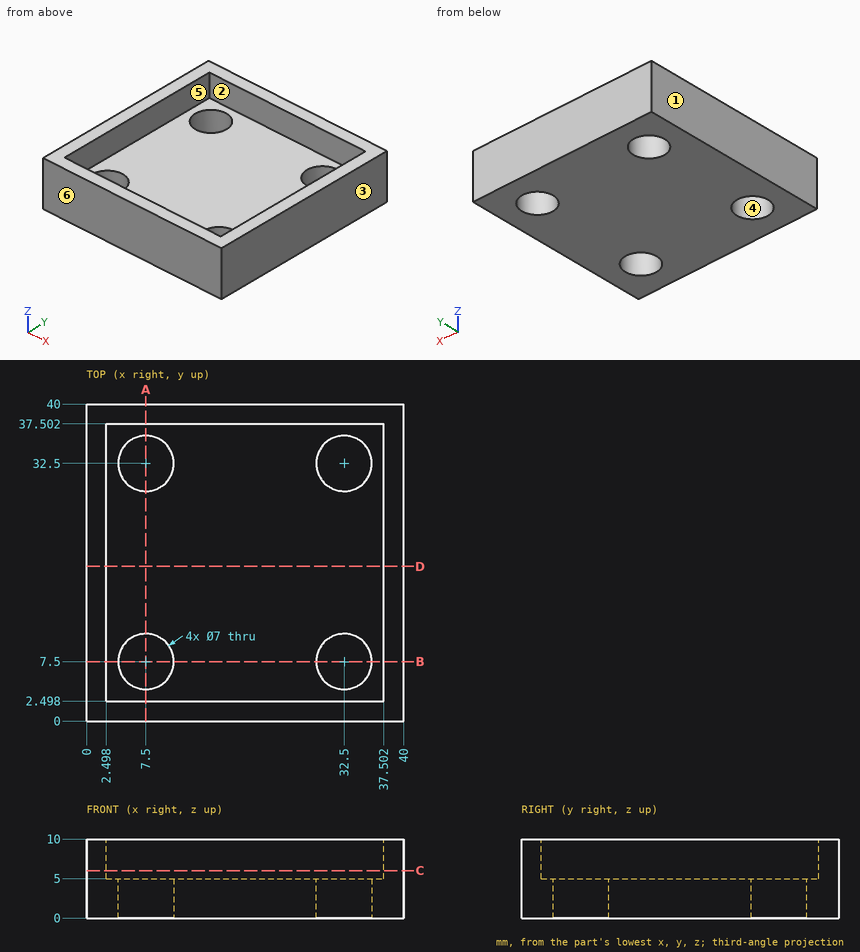
Job drawing, mm, ordinate dimensions from the low corner. One solid piece. A direction names the side the tool comes from. Coordinates: 2 decimals unless noted, no trailing zeros. Write each loop counter-clockwise with the first axis right and the second up, starting at its lowest first coordinate (ties: lowest second). Pieces come first, ordered by that corner, then holes. Notation, with made-up numbers: M -5.75,67.5 L 20.25,67.5 A9 ccw 20.25,72.5 Z; hole C 80.25,30 d6. An arc over 180 degrees is marked long. Answer as a JSON object with one key per item and string values. Group by question number.
1) Saw through at D-D (y = 19.5). Write the cut outline in (x, z), plus the area to 3 significant figures.
2) Saw through at A-A (x = 7.5). Write the cut outline in (y, z), plus the area to 3 significant figures.
3) Saw through at C-C (z = 6). Write the cut outline in (x, y).
4) Mould opens along X. For the marked faces 1, 2, 3 and 4 say: +X half, -X half, draft (parallel to the pull), parting line (faces both ways), or undercut.
5) Pin check, flat tips, straight feed: pin 1 Ø11 at (x, y) = (7.5, 32.5) entering from -Z; pin 2 Ø3 at (x, y) = (17, 30) entering from +Z; pin 3 Ø6.5 at (x, y) = (7.5, 7.5) entering from -Z. Stop position of each tip, or through.
6) Tool access for the marked faces 5 and 6: list every direction of +Z, -Z, +X, -X, +Y, -Y with a clear straight run to the whole face (end or side of a thin tool).
7) Wall check: line 1 (Y direction, x = 7.5, z = 3.45); line 2 (X direction, y = 31.5, z = 4); line 3 (X direction, y = 12, z = 9.25). Give the ranges that are in metal, low to high. Write a range as from..to.
Values follow:
{
 "1": {"outline": "M 0,0 L 40,0 L 40,10 L 37.5,10 L 37.5,5 L 2.5,5 L 2.5,10 L 0,10 Z", "area": "225 mm2"},
 "2": {"outline": "M 0,0 L 4,0 L 4,5 L 2.5,5 L 2.5,10 L 0,10 Z; M 11,0 L 29,0 L 29,5 L 11,5 Z; M 36,0 L 40,0 L 40,10 L 37.5,10 L 37.5,5 L 36,5 Z", "area": "155 mm2"},
 "3": {"outline": "M 0,0 L 40,0 L 40,40 L 0,40 Z; hole M 2.5,2.5 L 37.5,2.5 L 37.5,37.5 L 2.5,37.5 Z"},
 "4": {"face 1": "-X half", "face 2": "undercut", "face 3": "+X half", "face 4": "undercut"},
 "5": {"pin 1": "stops at z = 0", "pin 2": "stops at z = 5", "pin 3": "passes through"},
 "6": {"face 5": "+Z", "face 6": "+Z, -Z, +X, -X, -Y"},
 "7": {"line 1": "y = 0..4, 11..29, 36..40", "line 2": "x = 0..4.15, 10.85..29.15, 35.85..40", "line 3": "x = 0..2.5, 37.5..40"}
}
